Geometry check sheet. Reference: the model listing, model coordinates, mm. Face numbers are marked on the shaded views. A direction names the side the tool comes from. Round coordinates to 2 decimals unless told otherwise and drop trailing zeros. Write each loop counter-clockwise with the first axis right and the second up, starting at its lowest first coordinate (ties: lowest second). Pieces come first, ordered by that corner, then holes. Notation, with made-up numbers: (-31, -13.75) - (-26, -13.75) arc R11 cw to (-26, -3.75) - close; hole circle Ø1 at (0.25, -22.5). An arc over 180 degrees is marked (long way). Return JSON: item names as keys, results as strings.
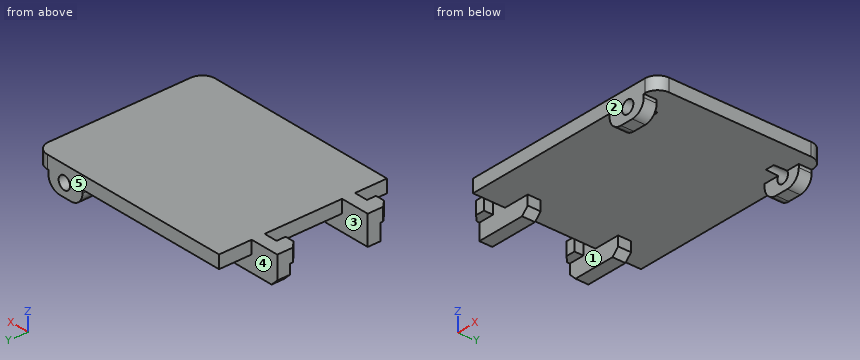
```python
from build123d import *

# Parameters (mm, degrees)
SKETCH_2_W          = 32.183544672
SKETCH_2_H          = 26
EXTRUDE_1_DEPTH     = 2
FILLET_1_R          = 2
SKETCH_5_W          = 6
SKETCH_5_H          = 2
EXTRUDE_2_DEPTH     = 2.5
FILLET_2_R          = 2
SKETCH_6_R          = 1
CUT_EXTRUDE_3_DEPTH = 4
CUT_EXTRUDE_3_TAPER = 2
SKETCH_7_R          = 1
CUT_EXTRUDE_4_DEPTH = 4
CUT_EXTRUDE_4_TAPER = 2
SKETCH_9_W          = 4.5
SKETCH_9_H          = 2
EXTRUDE_3_DEPTH     = 2
SKETCH_10_W         = 2.4
SKETCH_10_H         = 1.4
EXTRUDE_4_DEPTH     = 2
CHAMFER_1_SIZE      = 1
SKETCH_11_W         = 8.5
SKETCH_11_H         = 2
EXTRUDE_5_DEPTH     = 2.5
CHAMFER_2_SIZE      = 1


with BuildPart() as part:
    # 草图2 → 凸台-拉伸1 (new body)
    with BuildSketch(Plane.XY):
        with Locations((-0.901029093, -19.434236018)):
            Rectangle(SKETCH_2_W, SKETCH_2_H)
    extrude(amount=EXTRUDE_1_DEPTH)

    # 圆角1
    fillet_1_edges = [part.edges().sort_by_distance(p)[0] for p in [
        (15.190743243, -32.434236018, 1),
        (15.190743243, -6.434236018, 1),
    ]]
    fillet(fillet_1_edges, radius=FILLET_1_R)

    # 草图5 → 凸台-拉伸2 (add)
    with BuildSketch(Plane(origin=(0, 0, 0), x_dir=(-1, 0, 0), z_dir=(0, 0, -1))):
        with Locations((-10.007198571, -7.434236018)):
            Rectangle(SKETCH_5_W, SKETCH_5_H)
        with Locations((-10.007198571, -31.434236018)):
            Rectangle(SKETCH_5_W, SKETCH_5_H)
    extrude(amount=EXTRUDE_2_DEPTH)

    # 圆角2
    fillet_2_edges = [part.edges().sort_by_distance(p)[0] for p in [
        (13.007198571, -7.434236018, -2.5),
        (7.007198571, -7.434236018, -2.5),
        (13.007198571, -31.434236018, -2.5),
        (7.007198571, -31.434236018, -2.5),
    ]]
    fillet(fillet_2_edges, radius=FILLET_2_R)

    # 草图6 → 切除-拉伸3 (cut)
    with BuildSketch(Plane.XZ.offset(32.434236018)):
        with Locations((10.190743244, -0.5)):
            Circle(SKETCH_6_R)
    extrude(amount=-CUT_EXTRUDE_3_DEPTH, taper=CUT_EXTRUDE_3_TAPER, mode=Mode.SUBTRACT)

    # 草图7 → 切除-拉伸4 (cut)
    with BuildSketch(Plane(origin=(0, -6.434236018, 0), x_dir=(1, 0, 0), z_dir=(0, 1, 0))):
        with Locations((10.190743243, 0.5)):
            Circle(SKETCH_7_R)
    extrude(amount=-CUT_EXTRUDE_4_DEPTH, taper=CUT_EXTRUDE_4_TAPER, mode=Mode.SUBTRACT)

    # 草图9 → 凸台-拉伸3 (add)
    with BuildSketch(Plane(origin=(0, 0, 0), x_dir=(-1, 0, 0), z_dir=(0, 0, -1))):
        with Locations((19.242801429, -12.484236018)):
            Rectangle(SKETCH_9_W, SKETCH_9_H)
        with Locations((19.242801429, -26.484236018)):
            Rectangle(SKETCH_9_W, SKETCH_9_H)
    extrude(amount=-EXTRUDE_3_DEPTH)

    # 草图10 → 凸台-拉伸4 (add)
    with BuildSketch(Plane(origin=(0, 0, 0), x_dir=(-1, 0, 0), z_dir=(0, 0, -1))):
        with Locations((20.292801429, -14.184236018)):
            Rectangle(SKETCH_10_W, SKETCH_10_H)
        with Locations((20.292801429, -28.184236018)):
            Rectangle(SKETCH_10_W, SKETCH_10_H)
    extrude(amount=-EXTRUDE_4_DEPTH)

    # 倒角1
    chamfer_1_edges = [part.edges().sort_by_distance(p)[0] for p in [
        (-21.492801429, -14.884236018, 1),
        (-21.492801429, -28.884236018, 1),
    ]]
    chamfer(chamfer_1_edges, length=CHAMFER_1_SIZE)

    # 草图11 → 凸台-拉伸5 (add)
    with BuildSketch(Plane(origin=(0, 0, 0), x_dir=(-1, 0, 0), z_dir=(0, 0, -1))):
        with Locations((17.242801429, -12.484236018)):
            Rectangle(SKETCH_11_W, SKETCH_11_H)
        with Locations((17.242801429, -26.484236018)):
            Rectangle(SKETCH_11_W, SKETCH_11_H)
    extrude(amount=EXTRUDE_5_DEPTH)

    # 倒角2
    chamfer_2_edges = [part.edges().sort_by_distance(p)[0] for p in [
        (-21.492801429, -12.484236018, -2.5),
        (-12.992801429, -12.484236018, -2.5),
        (-12.992801429, -26.484236018, -2.5),
    ]]
    chamfer(chamfer_2_edges, length=CHAMFER_2_SIZE)


solid = part.part
```
(1) Section check C-C, the plane x = 12.5. Enter the section's corners in (y, z), plus the area to 3 significant figures.
Response values:
{"outline": "(-32.43, -1.83) - (-30.43, -1.83) - (-30.43, 0) - (-8.43, 0) - (-8.43, -1.83) - (-6.43, -1.83) - (-6.43, 2) - (-32.43, 2) - close", "area": "59.3 mm^2"}
(2) Material ranges on line 1 along Y through (x, z) = (-18, 1.4); line 2 along Z through (x, y) = (4, -11); line 3 along X through (y, z) = (-30, 0.75), recorded low to high. Write a range as [from, to].
Response values:
{"line 1": "y = [-27.48, -25.48], [-13.48, -11.48]", "line 2": "z = [0, 2]", "line 3": "x = [-16.99, 15.19]"}
(3) Section check B-B, the plane y = -26.5. Enter the section's corners in (x, z).
Response values:
{"outline": "(-21.49, -2.5) - (-13.99, -2.5) - (-12.99, -1.5) - (-12.99, 0) - (15.19, 0) - (15.19, 2) - (-21.49, 2) - close"}
(4) Gauge pin test, flat ends, axial feed: pin 1 (1 mm diameter, centred on x = -17, z = -1, fed in from +Y); pin 2 (1.1 mm diameter, centred on x = -19.5, z = 1.5, fed in from -Y); pin 3 (1 mm diameter, centred on x = 7.5, y = -21, fed in from -Z); pin 4 (1.3 mm diameter, centred on x = 11, z = -1, fed in from -Y). Record the tip position at first contact, or that the pin passes through.
Response values:
{"pin 1": "stops at y = -11.48", "pin 2": "stops at y = -28.88", "pin 3": "stops at z = 0", "pin 4": "stops at y = -32.43"}
(5) Access from +Z, -Z, +X, -X, +Y, -Y to the whole of each face (thin tool, end or side, straight path). Record for the marked faces 3, 4 and 5.
Response values:
{"face 3": "-Z, -X", "face 4": "-Z, -X, +Y", "face 5": "+Z, -Z, +X, -X, +Y"}
(6) Section check D-D, the plane z = -1.1. Give the number of separate pieces and of enclosed holes in the cut face, plus the area to 3 significant figures.
Response values:
{"separate pieces": "6", "enclosed holes": "0", "area": "51.2 mm^2"}
(7) Release check for a two-part mould opening along X. For the marked faces 1 and 2 record: pulls with the +X half, pulls with the -X half, needs draft (parallel to the pull), parting line crosses it, or undercut.
Response values:
{"face 1": "undercut", "face 2": "needs draft"}
(8) Section check A-A, the plane z = 1.55. Enter the section's corners in (x, y), plus the area to 3 significant figures.
Response values:
{"outline": "(-21.49, -27.88) - (-20.49, -28.88) - (-19.09, -28.88) - (-19.09, -27.48) - (-16.99, -27.48) - (-16.99, -32.43) - (13.19, -32.43) arc R2 ccw to (15.19, -30.43) - (15.19, -8.43) arc R2 ccw to (13.19, -6.43) - (-16.99, -6.43) - (-16.99, -11.48) - (-21.49, -11.48) - (-21.49, -13.88) - (-20.49, -14.88) - (-19.09, -14.88) - (-19.09, -13.48) - (-16.99, -13.48) - (-16.99, -25.48) - (-21.49, -25.48) - close", "area": "859 mm^2"}
